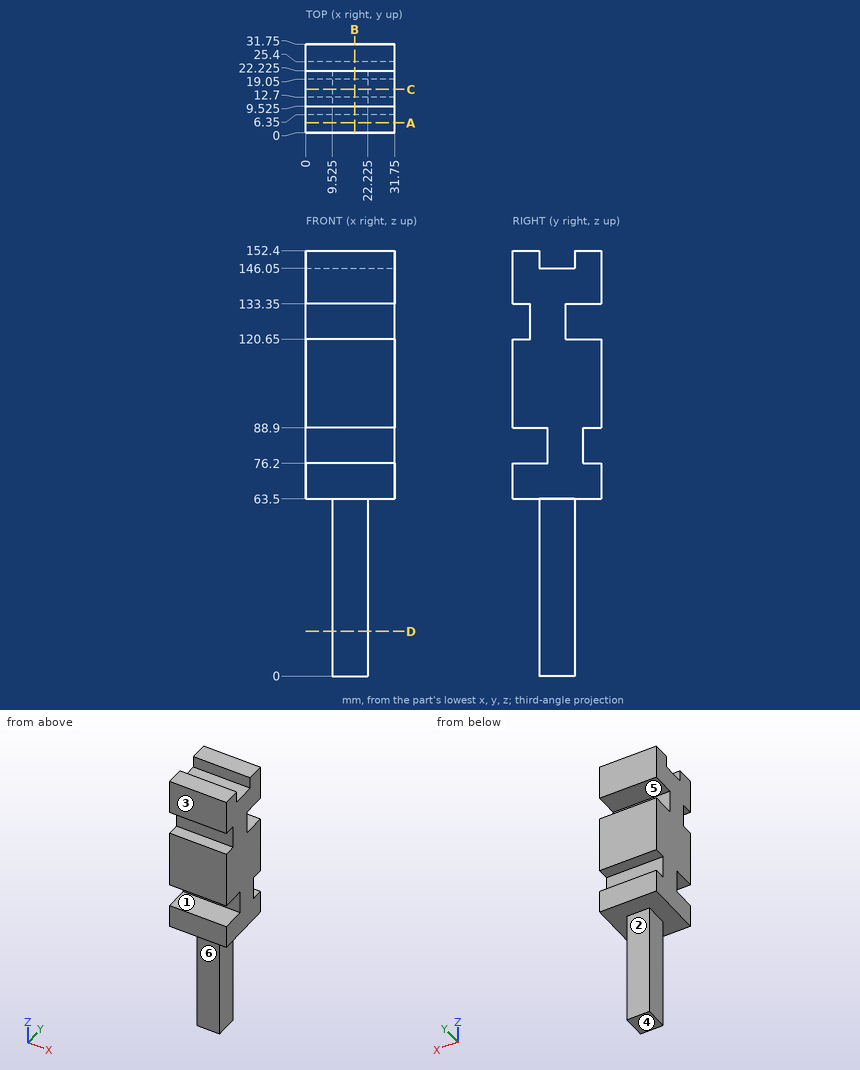
Check sheet for the drawn part. Datum: minimum x, y, z corner. Units: mm. A direction names the side the tool comes from. Round coordinates to 2 decimals unless told otherwise and drop trailing zeros. Loops run counter-clockwise (first coordinate to the right, second up) from the corner with the lowest first, then second, coordinate; pieces in that order, holes last.
Item 1: Mould release check, pull along Z, two halves, no side actions. Record for the marked faces 4, 5 and 6: pulls with the +Z half, pulls with the -Z half, needs draft (parallel to the pull), parting line crosses it, or undercut.
Item 2: Cross-section at C-C on y = 15.5. Record the boundary of the cut face in (x, z) (3 decimals), then the cut area to 3 significant figures.
Item 3: Access from +Z, -Z, +X, -X, +Y, -Y to the whole of each face (thin tool, end or side, straight path). Record for the marked faces 1, 2 and 3.
Item 4: Thickness scan on line 1 (Z direction, x = 7.5, y = 30.5); line 2 (Z direction, x = 20.5, y = 7); line 3 (Z direction, x = 19.5, y = 10). Record the ranges inside material, lowest first.
Item 5: Gauge pin test, flat ends, axial feed: pin 1 (1 mm diameter, centred on y = 9.5, z = 56.5, fed in from +X) (3 decimals); pin 2 (4 mm diameter, centred on x = 14.5, z = 127.5, fed in from +Y); pin 3 (14 mm diameter, centred on y = 15, z = 27.5, fed in from -X) (3 decimals). Record the tip position at first contact, or that the pin passes through.
Item 6: Cross-section at D-D on z = 16. Record the boundary of the cut face in (x, y) (3 decimals), then the cut area to 3 significant figures.
Item 7: Cross-section at B-B on x = 17.5. Record the boundary of the cut face in (y, z) (3 decimals), then the cut area to 3 significant figures.
Item 8: Cross-section at A-A on y = 3.5. Record the boundary of the cut face in (x, z).
Answer sheet:
1. face 4: pulls with the -Z half
1. face 5: undercut
1. face 6: needs draft
2. outline: (0, 63.5) - (9.525, 63.5) - (9.525, 0) - (22.225, 0) - (22.225, 63.5) - (31.75, 63.5) - (31.75, 146.05) - (0, 146.05) - close
2. area: 3,430 mm2
3. face 1: +X, -X, -Y
3. face 2: -Z, +X, -X, +Y
3. face 3: +Z, -Z, +X, -X, -Y
4. line 1: z = 63.5 to 76.2, 88.9 to 120.65, 133.35 to 152.4
4. line 2: z = 63.5 to 76.2, 88.9 to 152.4
4. line 3: z = 0 to 76.2, 88.9 to 146.05
5. pin 1: stops at x = 22.225
5. pin 2: stops at y = 19.05
5. pin 3: stops at x = 9.525
6. outline: (9.525, 9.525) - (22.225, 9.525) - (22.225, 22.225) - (9.525, 22.225) - close
6. area: 161 mm2
7. outline: (0, 63.5) - (9.525, 63.5) - (9.525, 0) - (22.225, 0) - (22.225, 63.5) - (31.75, 63.5) - (31.75, 76.2) - (25.4, 76.2) - (25.4, 88.9) - (31.75, 88.9) - (31.75, 120.65) - (19.05, 120.65) - (19.05, 133.35) - (31.75, 133.35) - (31.75, 152.4) - (22.225, 152.4) - (22.225, 146.05) - (9.525, 146.05) - (9.525, 152.4) - (0, 152.4) - (0, 133.35) - (6.35, 133.35) - (6.35, 120.65) - (0, 120.65) - (0, 88.9) - (12.7, 88.9) - (12.7, 76.2) - (0, 76.2) - close
7. area: 3,060 mm2
8. outline: (0, 63.5) - (31.75, 63.5) - (31.75, 76.2) - (0, 76.2) - close; (0, 88.9) - (31.75, 88.9) - (31.75, 120.65) - (0, 120.65) - close; (0, 133.35) - (31.75, 133.35) - (31.75, 152.4) - (0, 152.4) - close
